Geometry: final body of the model. Coordinates: model frame, mm. Coordinates: 2 decimals unless noted, no trailing zeros. Order: outer loops, then holes, each group sorted by start corner. A loop starts at its lowest first (then second) coordinate and runs counter-clockwise, first axis right, second up. Notation, with made-up numbers: (24, 64) - (42, 64) arc R15 cw to (42, 86) - close; hole circle Ø8 at (-20.5, 81.25). An arc over 180 degrees is marked (long way). Use one line per item in the form item = value. Start each with the question number.
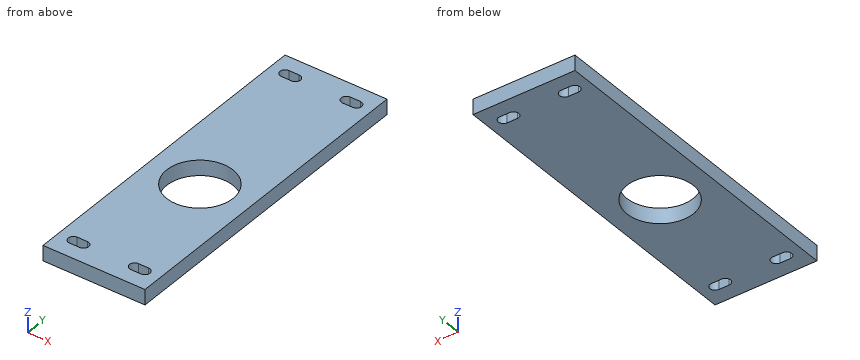
```python
from build123d import *

# Parameters (mm, degrees)
SKETCH1_W            = 63.5
SKETCH1_H            = 203.2
BOSS_EXTRUDE1_DEPTH  = 9.525
CUT_EXTRUDE1_DEPTH   = 107.870707516
LPATTERN1_COUNT      = 2
LPATTERN1_PITCH      = 38.1
LPATTERN1_COUNT_DIR2 = 2
LPATTERN1_PITCH_DIR2 = 177.8
SKETCH3_R            = 20.6375
CUT_EXTRUDE2_DEPTH   = 107.870707516


with BuildPart() as part:
    # Sketch1 → Boss-Extrude1 (new body)
    with BuildSketch(Plane.XY):
        Rectangle(SKETCH1_W, SKETCH1_H)
    extrude(amount=BOSS_EXTRUDE1_DEPTH)

    # Sketch2 → Cut-Extrude1 (cut, through all)
    with BuildSketch(Plane.XY.offset(9.525)):
        with BuildLine():
            Line((-22.225, 92.075), (-15.875, 92.075))
            ThreePointArc((-15.875, 92.075), (-12.7, 88.9), (-15.875, 85.725))
            Line((-15.875, 85.725), (-22.225, 85.725))
            ThreePointArc((-22.225, 85.725), (-25.4, 88.9), (-22.225, 92.075))
        make_face()
    cut_extrude1 = extrude(amount=-CUT_EXTRUDE1_DEPTH, mode=Mode.SUBTRACT)

    # LPattern1: Cut-Extrude1 2 × 2
    with Locations(*[(i * LPATTERN1_PITCH, -j * LPATTERN1_PITCH_DIR2, 0) for i in range(LPATTERN1_COUNT) for j in range(LPATTERN1_COUNT_DIR2) if (i, j) != (0, 0)]):
        add(cut_extrude1, mode=Mode.SUBTRACT)

    # Sketch3 → Cut-Extrude2 (cut, through all)
    with BuildSketch(Plane.XY.offset(9.525)):
        with Locations((0, -12.7)):
            Circle(SKETCH3_R)
    extrude(amount=-CUT_EXTRUDE2_DEPTH, mode=Mode.SUBTRACT)


solid = part.part
```
(1) Material intervals for L1, parallel to X at y = -13.5, z = 7.25; L2, parallel to Y at x = 0, z = 5.75; L3, parallel to Y at x = -16, z = 4.5 (3 decimals), sorted ascending. Write a range as from..to.
(2) Contact query for a flat-ended pin moving along its axis: pin 1 Ø25 at (x, y) = (0, -12.7) entering from +Z. Output: stop coordinate, or through.
(3) Cut plane C-C on x = 0. Return the cut outline in (y, z) (1 decimal), plus the area to 3 significant figures.
(4) Cut plane D-D on z = 6.25. Count the separate pieces of the cut face and the enclosed holes in it, plus the area to 3 significant figures.
(5) Cut plane B-B on y = 88.9. Return the cut outline in (x, z) (3 decimals), plus the area to 3 significant figures.
Check sheet entries:
q1.L1 = -31.75..-20.62, 20.62..31.75
q1.L2 = -101.6..-33.34, 7.94..101.6
q1.L3 = -101.6..-92.075, -85.725..-25.735, 0.335..85.725, 92.075..101.6
q2.pin_1 = through
q3.outline = (-101.6, 0) - (-33.3, 0) - (-33.3, 9.5) - (-101.6, 9.5) - close; (7.9, 0) - (101.6, 0) - (101.6, 9.5) - (7.9, 9.5) - close
q3.area = 1,540 mm^2
q4.separate_pieces = 1
q4.enclosed_holes = 5
q4.area = 11,300 mm^2
q5.outline = (-31.75, 0) - (-25.4, 0) - (-25.4, 9.525) - (-31.75, 9.525) - close; (-12.7, 0) - (12.7, 0) - (12.7, 9.525) - (-12.7, 9.525) - close; (25.4, 0) - (31.75, 0) - (31.75, 9.525) - (25.4, 9.525) - close
q5.area = 363 mm^2
